Input: part model. Units: mm. Frame: model coordinates. Face numbers are marked on the shaded views. A direction names the side the tool comes from. Give positions to 0.01 mm unless a question says otherwise; leave off trailing zeros. Loops run counter-clockwise (first coordinate to the right, second up) from the corner with the lowest first, then second, coordinate; pieces in that order, holes last. Notation, with made-up numbers: (-7.5, -22) -> (9.5, -22) arc R21 ccw to (9.5, 13) -> close; hole circle Ø4 at (54, 75.25). An arc over 180 degrees is marked (long way). One line per question, with ' | ' between items.
from build123d import *
from build123d.topology import SkipClean

# Parameters (mm, degrees)
SKETCH1_R           = 2.75
BOSS_EXTRUDE1_DEPTH = 1.8
BOSS_EXTRUDE2_DEPTH = 21.7
SKETCH4_R           = 6
BOSS_EXTRUDE3_DEPTH = 10
BOSS_EXTRUDE4_START = 18
SKETCH5_R           = 6
SKETCH5_R_2         = 4.9
BOSS_EXTRUDE4_DEPTH = 18


with BuildPart() as part:
    # Sketch1 → Boss-Extrude1 (new body)
    with BuildSketch(Plane(origin=(0, 0, 0), x_dir=(1, 0, 0), z_dir=(0, 1, 0))):
        with Locations(Location((0, 0, 0), (0, 0, 270))):
            Circle(SKETCH1_R)
    extrude(amount=BOSS_EXTRUDE1_DEPTH)

    # Sketch3 → Boss-Extrude2 (add)
    with SkipClean():  # the faces are left unmerged after this step: merging them gives an invalid solid
        with BuildSketch(Plane(origin=(0, 1.8, 0), x_dir=(1, 0, 0), z_dir=(0, 1, 0))):
            with BuildLine():
                Line((-2.0790623, 1.799999987), (2.0790623, 1.799999987))
                ThreePointArc((2.0790623, 1.799999987), (2.75, 0), (2.0790623, -1.799999987))
                Line((2.0790623, -1.799999987), (-2.0790623, -1.799999987))
                ThreePointArc((-2.0790623, -1.799999987), (-2.75, 0), (-2.0790623, 1.799999987))
            make_face()
        extrude(amount=BOSS_EXTRUDE2_DEPTH)

    # Sketch4 → Boss-Extrude3 (add)
    with SkipClean():  # the faces are left unmerged after this step: merging them gives an invalid solid
        with BuildSketch(Plane.XZ):
            with Locations(Location((0, 0, 0), (0, 0, 270))):
                Circle(SKETCH4_R)
        extrude(amount=BOSS_EXTRUDE3_DEPTH)

    # Sketch5 → Boss-Extrude4 (add)
    with BuildSketch(Plane(origin=(0, 0, 0), x_dir=(1, 0, 0), z_dir=(0, 1, 0)).offset(BOSS_EXTRUDE4_START)):
        with Locations(Location((0, 0, 0), (0, 0, 270))):
            Circle(SKETCH5_R)
        with Locations(Location((0, 0, 0), (0, 0, 270))):
            Circle(SKETCH5_R_2, mode=Mode.SUBTRACT)
    extrude(amount=-BOSS_EXTRUDE4_DEPTH)


solid = part.part
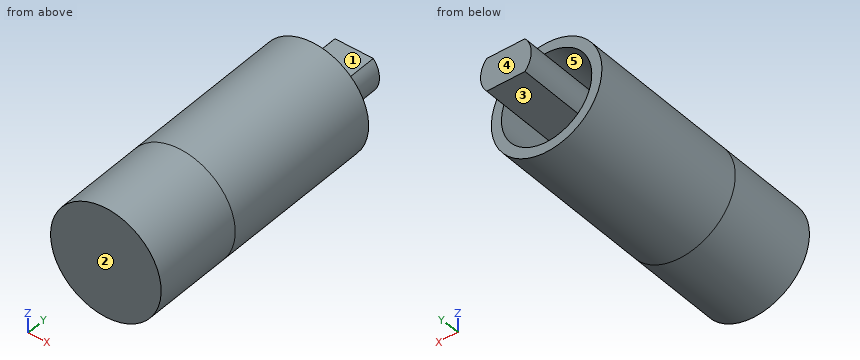
1. Pull-direction query (Z, two-part tool) for the marked faces 1, 2 and 3; classes: pulls with the +Z half, pulls with the -Z half, needs draft (parallel to the pull), parting line crosses it, or undercut.
Determined:
face 1: undercut | face 2: needs draft | face 3: undercut
2. Section query A-A (x = 0). Output: boundary loops of the cut face in (y, z), then the cut area to 3 significant figures.
Determined:
outline: (-10, -6) -> (18, -6) -> (18, -4.9) -> (0, -4.9) -> (0, -2.75) -> (1.8, -2.75) -> (1.8, -1.8) -> (23.5, -1.8) -> (23.5, 1.8) -> (1.8, 1.8) -> (1.8, 2.75) -> (0, 2.75) -> (0, 4.9) -> (18, 4.9) -> (18, 6) -> (-10, 6) -> close | area: 248 mm2
3. Section query D-D (z = -4.25). Output: boundary loops of the cut face in (x, y).
Determined:
outline: (-4.24, -10) -> (4.24, -10) -> (4.24, 18) -> (2.44, 18) -> (2.44, 0) -> (-2.44, 0) -> (-2.44, 18) -> (-4.24, 18) -> close
4. Reachability of the marked faces 4 and 5 from +Z, -Z, +X, -X, +Y, -Y: full face, straight path, thin tool, end or side. Return the list, or none.
Determined:
face 4: +Z, -Z, +X, -X, +Y | face 5: +Y
5. Ray query, line 1 along Z through (x, y) = (-0.5, 1.5); line 2 along Z through (x, y) = (-1.75, 16); line 3 along Y through (x, z) = (2.5, -3.5). Return the intervals inside material, ascending. Write a range as from..to.
Determined:
line 1: z = -5.98..-4.87, -2.7..2.7, 4.87..5.98 | line 2: z = -5.74..-4.58, -1.8..1.8, 4.58..5.74 | line 3: y = -10..0
6. Section query B-B (z = 0). Output: boundary loops of the cut face in (x, y), then the cut area to 3 significant figures.
Determined:
outline: (-6, -10) -> (6, -10) -> (6, 18) -> (4.9, 18) -> (4.9, 0) -> (2.75, 0) -> (2.75, 23.5) -> (-2.75, 23.5) -> (-2.75, 0) -> (-4.9, 0) -> (-4.9, 18) -> (-6, 18) -> close | area: 289 mm2
7. Pin query (flat end, axial travel): P1, Ø1, axis at x = 1, z = 2.5, coming from the +Y side; P2, Ø1, axis at x = 3, y = 3.5, coming from the +Z side. Return the tip coordinate at first contact, or that it passes through.
Determined:
P1: stops at y = 1.8 | P2: stops at z = 5.45
8. Section query C-C (y = -6.5). Output: boundary loops of the cut face in (x, z).
Determined:
outline: circle Ø12 at (0, 0)
